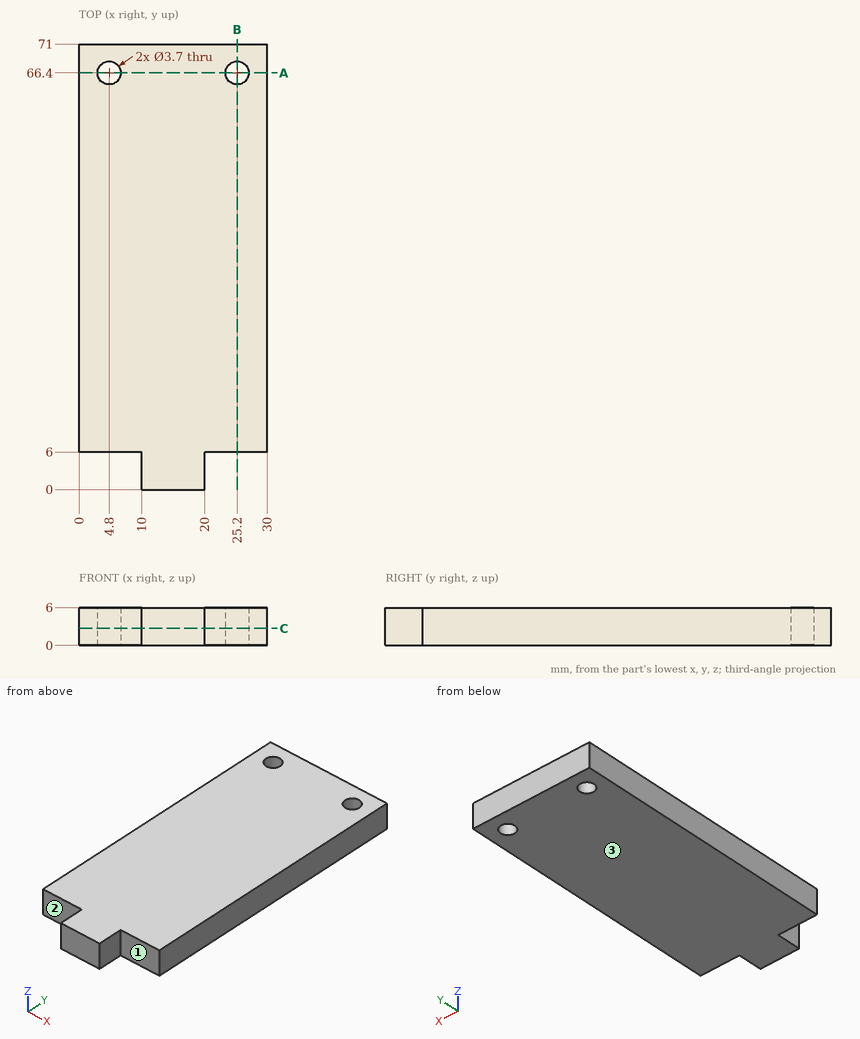
Design review of the part shown in the three views and the two pictorial views. Dimensions are in mm from the part's minimum x, y and z. A direction names the side the tool comes from. Coordinates: 2 decimals unless noted, no trailing zeros. Loops run counter-clockwise (first coordinate to the right, second up) from the corner with the lowest first, then second, coordinate; pieces in that order, holes last. Notation, with made-up numbers: (54, 75) -> (67, 75) arc R16 ccw to (67, 84) -> close; hole circle Ø2 at (18.25, 86). An arc over 180 degrees is marked (long way). Answer as CSV lines item,"result".
Item 1: Insertion check: pin 1 (1.5 mm diameter, centred on x = 15.5, z = 1, fed in from -Y); pin 2 (3 mm diameter, centred on y = 2, z = 3, fed in from -X); pin 3 (3 mm diameter, centred on x = 7.5, z = 5, fed in from -Y). Each pin has a flat end and moves straight along its axis. Give the tip position at first contact, or say it passes through.
Results below:
pin 1,"stops at y = 0"
pin 2,"stops at x = 10"
pin 3,"stops at y = 6"
Item 2: Machinability: for the marked faces 1, 2 and 3, which of the approach directions +Z, -Z, +X, -X, +Y, -Y give a long, thin tool a straight path to every point of the face, cutting with its end or side? Answer none if there is none.
Results below:
face 1,"+Z, -Z, +X, -Y"
face 2,"+Z, -Z, -X, -Y"
face 3,"-Z, +X, -X, +Y, -Y"
Item 3: Take a section at A-A, the plane y = 66.4. State the section outline as (x, z) points.
Results below:
outline,"(0, 0) -> (2.95, 0) -> (2.95, 6) -> (0, 6) -> close; (6.65, 0) -> (23.35, 0) -> (23.35, 6) -> (6.65, 6) -> close; (27.05, 0) -> (30, 0) -> (30, 6) -> (27.05, 6) -> close"
Item 4: For L1, parallel to X at y = 66.4, z = 2.65; L2, parallel to Y at x = 25.2, z = 4.5; L3, parallel to Y at x = 7, z = 3.2, list the stretches that pass through material, from the lowest coordinate up.
Results below:
L1,"x = 0 to 2.95, 6.65 to 23.35, 27.05 to 30"
L2,"y = 6 to 64.55, 68.25 to 71"
L3,"y = 6 to 71"
Item 5: Take a section at C-C, the plane z = 2.7. State the section outline as (x, y) points.
Results below:
outline,"(0, 6) -> (10, 6) -> (10, 0) -> (20, 0) -> (20, 6) -> (30, 6) -> (30, 71) -> (0, 71) -> close; hole circle Ø3.7 at (4.8, 66.4); hole circle Ø3.7 at (25.2, 66.4)"
Item 6: Take a section at B-B, the plane x = 25.2. State the section outline as (y, z) points.
Results below:
outline,"(6, 0) -> (64.55, 0) -> (64.55, 6) -> (6, 6) -> close; (68.25, 0) -> (71, 0) -> (71, 6) -> (68.25, 6) -> close"
